Geometry check sheet. Reference: the model listing, model coordinates, mm. Face numbers are marked on the shaded views. A direction names the side the tool comes from. Round coordinates to 2 decimals unless told otherwise and drop trailing zeros. Write each loop counter-clockwise with the first axis right and the second up, starting at its lowest first coordinate (ties: lowest second). Pieces come first, ordered by that corner, then holes. Notation, with made-up numbers: M 51.25,-18 L 95.25,-18 A30 cw 95.25,9 Z; hole C 33.5,26.25 d6. An arc over 180 degrees is marked long. Put each result on its own line as item: value. Start each with the question number.
(1) Section check A-A on x = 19. Record the cut outline in (y, z) (3 decimals).
(2) Gauge pin test, flat ends, axial feed: pin 1 (4.5 mm diameter, centred on x = 20.5, y = 19, fed in from -Z); pin 2 (12 mm diameter, centred on x = 28, z = -2.5, fed in from +Y); pin 3 (7.5 mm diameter, centred on x = 22, z = -2, fed in from -Y). Record the tip position at first contact, or that the pin passes through.
(3) Section check C-C on x = 33. Record the cut outline in (y, z), then the cut area to 3 significant figures.
(4) Section check D-D on z = 22. Record the cut outline in (x, y) (3 decimals).
(5) Tool access check on the marked faces 4, 5, 6 and 7. Record the directions out of +Z, -Z, +X, -X, +Y, -Y that give a thin tool (end or side, any length) a straight path to the whole face; none if there is none.
(6) Material ranges on probe 1 along Y at (x, z) = (19, -4); probe 2 along X at (y, z) = (27, -5); probe 3 along Y at (x, z) = (7.5, 8.5), recorded low to high.
(7) Mould release check, pull along Z, two halves, no side actions. Record for the marked faces 1, 2 and 3: pulls with the +Z half, pulls with the -Z half, needs draft (parallel to the pull), parting line crosses it, or undercut.
(8) Section check B-B on z = -10. Record the cut outline in (x, y).
from build123d import *

# Parameters (mm, degrees)
BOSS_EXTRUDE1_DEPTH = 38
BOSS_EXTRUDE2_DEPTH = 14
SKETCH3_R           = 15.81
CUT_EXTRUDE1_DEPTH  = 67.258961658
BOSS_EXTRUDE3_DEPTH = 8
SKETCH5_R           = 2.875
BOSS_EXTRUDE4_DEPTH = 14


with BuildPart() as part:
    # Sketch1 → Boss-Extrude1 (new body)
    with BuildSketch(Plane(origin=(0, 0, 0), x_dir=(0, 0, -1), z_dir=(1, 0, 0))):
        Polygon((-12.75, 0), (-12.75, 7), (12.75, 7), (12.75, 0), (14, 0), (14, 8.5), (-14, 8.5), (-14, 0), align=None)
    extrude(amount=BOSS_EXTRUDE1_DEPTH)

    # Sketch2 → Boss-Extrude2 (add, symmetric)
    with BuildSketch(Plane.XY):
        with BuildLine():
            Line((0, 27.5), (0, 8.5))
            Line((0, 8.5), (38, 8.5))
            Line((38, 8.5), (38, 27.5))
            ThreePointArc((38, 27.5), (19, 46.5), (0, 27.5))
        make_face()
    extrude(amount=BOSS_EXTRUDE2_DEPTH, both=True)

    # Sketch3 → Cut-Extrude1 (cut, through all)
    with BuildSketch(Plane.XY.offset(14)):
        with Locations((19, 27.5)):
            Circle(SKETCH3_R)
    extrude(amount=-CUT_EXTRUDE1_DEPTH, mode=Mode.SUBTRACT)

    # Sketch4 → Boss-Extrude3 (add)
    with BuildSketch(Plane.XY.offset(14)):
        with BuildLine():
            Line((21.925, 27.5), (21.925, 11.962932226))
            ThreePointArc((21.925, 11.962932226), (19, 11.69), (16.075, 11.962932226))
            Line((16.075, 11.962932226), (16.075, 27.5))
            ThreePointArc((16.075, 27.5), (19, 30.425), (21.925, 27.5))
        make_face()
    extrude(amount=-BOSS_EXTRUDE3_DEPTH)

    # Sketch5 → Boss-Extrude4 (add)
    with BuildSketch(Plane.XY.offset(14)):
        with Locations(Location((19, 27.5, 0), (0, 0, 180))):
            Circle(SKETCH5_R)
    extrude(amount=BOSS_EXTRUDE4_DEPTH)


solid = part.part
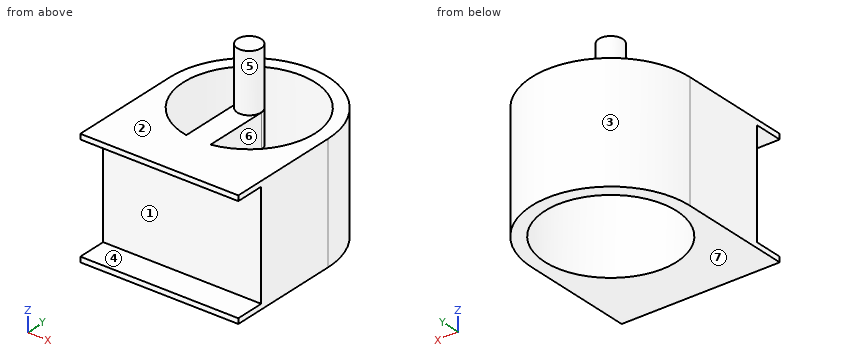
Answers follow:
1. outline: M 0,-14 L 11.69,-14 L 11.69,6 L 30.425,6 L 30.425,14 L 30.375,14 L 30.375,28 L 24.625,28 L 24.625,14 L 0,14 L 0,12.75 L 7,12.75 L 7,-12.75 L 0,-12.75 Z; M 43.31,-14 L 46.5,-14 L 46.5,14 L 43.31,14 Z
2. pin 1: stops at z = 6
2. pin 2: stops at y = 46.26
2. pin 3: stops at y = 7
3. outline: M 0,-14 L 20.15,-14 L 20.15,14 L 0,14 L 0,12.75 L 7,12.75 L 7,-12.75 L 0,-12.75 Z; M 34.85,-14 L 40.35,-14 L 40.35,14 L 34.85,14 Z
3. area: 540 mm^2
4. outline: C 19,27.5 d5.75
5. face 4: +X, -X, -Y
5. face 5: +Z
5. face 6: +Z, -Z
5. face 7: -Z, +X, -X, +Y, -Y
6. probe 1: y = 7 to 11.69, 43.31 to 46.5
6. probe 2: x = 0 to 3.2, 34.8 to 38
6. probe 3: y = 7 to 16.65, 38.35 to 42.62
7. face 1: undercut
7. face 2: pulls with the +Z half
7. face 3: needs draft
8. outline: M 0,7 L 38,7 L 38,27.5 A19 ccw 0,27.5 Z; hole C 19,27.5 d31.62
